Autodesk Inventor part; units mm, degrees
ref_plane "作業平面1" through (-9.5, -10, 1000) normal (0, 0, 1) x (1, 0, 0)
ref_plane "YZ Plane" through (0, 0, 0) normal (1, 0, 0) x (0, 1, 0)
ref_plane "XZ Plane" through (0, 0, 0) normal (0, 1, 0) x (-1, 0, 0)
ref_plane "作業平面1" through (-9.5, -10, 1000) normal (0, 0, 1) x (1, 0, 0)
sketch "スケッチ1" plane through (-9.5, -10, 1000) normal (0, 0, 1) x (1, 0, 0)
  line L0 (7.35, 18.5) -> (7.35, 20)
  line L1 (7.35, 20) -> (0, 20)
  arc A0 (0, 20) -> (-0.5, 19.5) centre (0, 19.5) ccw
  line L2 (-0.5, 19.5) -> (-0.5, 12.15)
  line L3 (-0.5, 12.15) -> (1, 12.15)
  line L4 (1, 12.15) -> (1, 14.15)
  line L5 (1, 14.15) -> (4.7, 14.15)
  line L6 (4.7, 14.15) -> (4.7, 12.15)
  line L7 (4.7, 12.15) -> (6.5, 12.15)
  line L8 (6.5, 12.15) -> (6.5, 7.85)
  line L9 (6.5, 7.85) -> (4.7, 7.85)
  line L10 (4.7, 7.85) -> (4.7, 5.85)
  line L11 (4.7, 5.85) -> (1, 5.85)
  line L12 (1, 5.85) -> (1, 7.85)
  line L13 (1, 7.85) -> (-0.5, 7.85)
  line L14 (-0.5, 7.85) -> (-0.5, 0.5)
  arc A1 (-0.5, 0.5) -> (0, 0) centre (0, 0.5) ccw
  line L15 (0, 0) -> (19, 0)
  arc A2 (19, 0) -> (19.5, 0.5) centre (19, 0.5) ccw
  line L16 (19.5, 0.5) -> (19.5, 7.85)
  line L17 (19.5, 7.85) -> (18, 7.85)
  line L18 (18, 7.85) -> (18, 5.85)
  line L19 (18, 5.85) -> (14.3, 5.85)
  line L20 (14.3, 5.85) -> (14.3, 7.85)
  line L21 (14.3, 7.85) -> (12.5, 7.85)
  line L22 (12.5, 7.85) -> (12.5, 12.15)
  line L23 (12.5, 12.15) -> (14.3, 12.15)
  line L24 (14.3, 12.15) -> (14.3, 14.15)
  line L25 (14.3, 14.15) -> (18, 14.15)
  line L26 (18, 14.15) -> (18, 12.15)
  line L27 (18, 12.15) -> (19.5, 12.15)
  line L28 (19.5, 12.15) -> (19.5, 19.5)
  arc A3 (19.5, 19.5) -> (19, 20) centre (19, 19.5) ccw
  line L29 (19, 20) -> (11.65, 20)
  line L30 (11.65, 20) -> (11.65, 18.5)
  line L31 (11.65, 18.5) -> (13.65, 18.5)
  line L32 (13.65, 18.5) -> (13.65, 14.8)
  line L33 (13.65, 14.8) -> (11.65, 14.8)
  line L34 (11.65, 14.8) -> (11.65, 13)
  line L35 (11.65, 13) -> (7.35, 13)
  line L36 (7.35, 13) -> (7.35, 14.8)
  line L37 (7.35, 14.8) -> (5.35, 14.8)
  line L38 (5.35, 14.8) -> (5.35, 18.5)
  line L39 (5.35, 18.5) -> (7.35, 18.5)
  arc A4 (11.6496, 6.4) -> (11.0496, 7) centre (11.0496, 6.4) ccw
  line L40 (11.6496, 6.4) -> (11.6496, 5.5)
  arc A5 (11.6496, 5.5) -> (11.9496, 5.2) centre (11.9496, 5.5) ccw
  line L41 (11.9496, 5.2) -> (13.3496, 5.2)
  arc A6 (13.6496, 4.9) -> (13.3496, 5.2) centre (13.3496, 4.9) ccw
  arc A7 (13.6496, 4.9) -> (13.7891, 4.5617) centre (13.9391, 4.8215) ccw
  line L42 (13.7891, 4.5617) -> (14.3769, 4.2223)
  arc A8 (14.3769, 4.2223) -> (15.0013, 4.3244) centre (14.6267, 4.6555) ccw
  arc A9 (15.0029, 1.6738) -> (15.0013, 4.3244) centre (16.5, 3) ccw
  arc A10 (15.0029, 1.6738) -> (14.3787, 1.7753) centre (14.6287, 1.3422) ccw
  line L43 (14.3787, 1.7753) -> (13.9715, 1.5402)
  arc A11 (13.8215, 1.5) -> (13.9715, 1.5402) centre (13.8215, 1.8) ccw
  line L44 (13.8215, 1.5) -> (5.1785, 1.5)
  arc A12 (5.0285, 1.5402) -> (5.1785, 1.5) centre (5.1785, 1.8) ccw
  line L45 (5.0285, 1.5402) -> (4.6213, 1.7753)
  arc A13 (4.6213, 1.7753) -> (3.9971, 1.6738) centre (4.3713, 1.3422) ccw
  arc A14 (3.9971, 4.3262) -> (3.9971, 1.6738) centre (2.5, 3) ccw
  arc A15 (3.9971, 4.3262) -> (4.6213, 4.2247) centre (4.3713, 4.6578) ccw
  line L46 (4.6213, 4.2247) -> (5.2, 4.5588)
  arc A16 (5.2, 4.5588) -> (5.35, 4.8187) centre (5.05, 4.8187) ccw
  arc A17 (5.6395, 5.1972) -> (5.35, 4.8187) centre (5.6395, 4.8972) ccw
  line L47 (5.6395, 5.1972) -> (7.05, 5.1972)
  arc A18 (7.05, 5.1972) -> (7.35, 5.4972) centre (7.05, 5.4972) ccw
  line L48 (7.35, 5.4972) -> (7.35, 6.4)
  arc A19 (7.95, 7) -> (7.35, 6.4) centre (7.95, 6.4) ccw
  line L49 (7.95, 7) -> (11.0496, 7)
  circle A20 centre (2.5, 17) radius 2
  circle A21 centre (16.5, 17) radius 2
  circle A22 centre (9.5, 10) radius 1.65
  point P0 (9.5, 10)
extrude "押し出し1" add sketch "スケッチ1" along normal blind 290
properties part number "AFSF-2020-4"
Read the model definition and answer for the solid it produces. Units are mm, in the model's axes. Give positions to 0.01 mm unless a question says otherwise; leave off trailing zeros. Write item = value, one per line.
1. Straight lines are drawn through the part: line 1 along Y through (x, z) = (-7, 1263.5); line 2 along Y through (x, z) = (4.5, 1043); line 3 along Y through (x, z) = (2.5, 1134.5). For each, find the intervals that lie inside material, in ascending order.
Numbers:
line_1 = -10 to -9, -5 to -4.15, 4.15 to 5, 9 to 10
line_2 = -10 to -8.44, -5.56 to -2.15, 2.15 to 10
line_3 = -10 to -8.5, -4.8 to 4.8, 8.5 to 10
2. Given pin 1 (3 mm diameter, centred on x = 0, z = 1214.5, fed in from +Y); pin 2 (2.5 mm diameter, centred on x = 7, y = 7, fed in from +Z), each flat-ended and moving along its own axis, determine where each tip first touches the part or whether it passes through.
Numbers:
pin_1 = 3
pin_2 = through
3. A cutting plane is placed at A-A, the plane z = 1036.5. Count the separate pieces of the cut face and the enclosed holes in it, and give its area (3 significant figures).
Numbers:
separate_pieces = 1
enclosed_holes = 4
area = 163 mm²
4. The mould has two halves that part along Y. Classify faces 1 (the face through (0, -8.5, 1143)), 2 (the face through (0, -10, 1143)), 3 (the face through (10, 6, 1143)): +Y half, -Y half, draft (parallel to the pull), parting line (faces both ways), or undercut.
Numbers:
face_1 = undercut
face_2 = -Y half
face_3 = draft
